Geometry: final body of the model. Coordinates: model frame, mm. A direction names the side the tool comes from. Round coordinates to 2 decimals unless told otherwise and drop trailing zeros. Loops run counter-clockwise (first coordinate to the right, second up) from the corner with the lowest first, then second, coordinate; pieces in that order, holes last. Notation, with made-up numbers: (86.25, 66.5) - (114.25, 66.5) arc R10 cw to (114.25, 70.5) - close; hole circle Ø7 at (78, 5.5). An arc over 180 degrees is marked (long way). Answer as a JSON object with one key per item and string values. Group by question number.
Item 1: Section A-A (z = 30.5). Return the cut outline in (x, y).
Item 2: Line query: line 1 (Y direction, x = 56, z = 1); line 2 (X direction, y = -19.5, z = 27.5); line 3 (Z direction, x = 37, y = 18.5). Output: solid intervals per line, ascending.
Item 3: Reachability of faces 5 (the face through (45, 0, 24)), 6 (the face through (-45, 0, 24)), 7 (the face through (40, 0, 24)) from +Z, -Z, +X, -X, +Y, -Y: full face, straight path, thin tool, end or side. Return the list, or none.
Item 4: Section B-B (x = 56.25). Return the cut outline in (y, z).
Item 5: Section D-D (y = -2.5). Return the cut outline in (x, z), plus the area to 3 significant figures.
Item 6: First-contact query: pin 1 (1 mm diameter, centred on x = 36.5, y = -1, fed in from +Z); pin 2 (4 mm diameter, centred on y = -10.5, z = 26.5, fed in from +X); pin 3 (6 mm diameter, centred on y = 4.5, z = 9.5, fed in from -X). Flat tips, straight axial feed; report the tip coordinate or a pass-through.
Item 7: Section C-C (y = 15). Return the cut outline in (x, z), plus the area to 3 significant figures.
Item 8: Draft query along Y for faces 1 (the face through (0, -22.5, 2)), 2 (the face through (-59, 0, 4)), 3 (the face through (0, 22.5, 2)), 4 (the face through (-59.3, 14.9, 2)). Return one class per face: released by +Y, released by -Y, zero draft, split by the parting line, or undercut.
Autodesk Inventor part; units mm, degrees
ref_plane "YZ Plane" through (0, 0, 0) normal (1, 0, 0) x (0, 1, 0)
ref_plane "XZ Plane" through (0, 0, 0) normal (0, 1, 0) x (-1, 0, 0)
ref_plane "XY Plane" through (0, 0, 0) normal (0, 0, 1) x (1, 0, 0)
sketch "Sketch1" plane through (0, 0, 0) normal (0, 0, 1) x (1, 0, 0)
  line L0 (-56.25, -15) -> (56.25, -15) construction
  line L1 (56.25, -15) -> (56.25, 15) construction
  line L2 (56.25, 15) -> (-56.25, 15) construction
  line L3 (-56.25, 15) -> (-56.25, -15) construction
  line L4 (-56.25, -15) -> (56.25, 15) construction
  line L5 (56.25, -15) -> (-56.25, 15) construction
  circle A0 centre (-56.25, 15) radius 3.05
  circle A1 centre (56.25, 15) radius 3.05
  circle A2 centre (56.25, -15) radius 3.05
  circle A3 centre (-56.25, -15) radius 3.05
  line L6 (-72.5, -22.5) -> (72.5, -22.5)
  line L7 (72.5, -22.5) -> (72.5, 22.5)
  line L8 (72.5, 22.5) -> (-72.5, 22.5)
  line L9 (-72.5, 22.5) -> (-72.5, -22.5)
  line L10 (-72.5, -22.5) -> (72.5, 22.5) construction
  line L11 (72.5, -22.5) -> (-72.5, 22.5) construction
  point P0 (0, 0)
  dimension "d0" = 112.5
  dimension "d1" = 30
  dimension "d2" = 6.1
  dimension "d3" = 145
  dimension "d4" = 45
extrude "Extrusion1" add sketch "Sketch1" along normal blind 4
sketch "Sketch2" plane through (0, 0, 4) normal (0, 0, 1) x (1, 0, 0)
  line L0 (72.5, 22.5) -> (-72.5, 22.5)
  line L1 (-72.5, -22.5) -> (72.5, -22.5)
  line L2 (-45, 22.5) -> (-40, 22.5)
  line L3 (-40, 22.5) -> (-40, -22.5)
  line L4 (-40, -22.5) -> (-45, -22.5)
  line L5 (-45, -22.5) -> (-45, 22.5)
  line L6 (40, 22.5) -> (45, 22.5)
  line L7 (45, 22.5) -> (45, -22.5)
  line L8 (45, -22.5) -> (40, -22.5)
  line L9 (40, -22.5) -> (40, 22.5)
  line L10 (-72.5, 22.5) -> (-72.5, -22.5)
  point P0 (0, 0)
  dimension "d7" = 5
  dimension "d8" = 5
  dimension "d9" = 80
  dimension "d10" = 27.5
extrude "Extrusion2" add sketch "Sketch2" along normal blind 40 contours L7 L1 L9 L0 | L3 L1 L5 L0
properties part number "WheelModuleBracket" material "ABS Plastic"
Values:
{
 "1": {"outline": "(-45, -22.5) - (-40, -22.5) - (-40, 22.5) - (-45, 22.5) - close; (40, -22.5) - (45, -22.5) - (45, 22.5) - (40, 22.5) - close"},
 "2": {"line 1": "y = -22.5 to -18.04, -11.96 to 11.96, 18.04 to 22.5", "line 2": "x = -45 to -40, 40 to 45", "line 3": "z = 0 to 4"},
 "3": {"face 5": "+Z, +X, +Y, -Y", "face 6": "+Z, -X, +Y, -Y", "face 7": "+Z, +Y, -Y"},
 "4": {"outline": "(-22.5, 0) - (-18.05, 0) - (-18.05, 4) - (-22.5, 4) - close; (-11.95, 0) - (11.95, 0) - (11.95, 4) - (-11.95, 4) - close; (18.05, 0) - (22.5, 0) - (22.5, 4) - (18.05, 4) - close"},
 "5": {"outline": "(-72.5, 0) - (72.5, 0) - (72.5, 4) - (45, 4) - (45, 44) - (40, 44) - (40, 4) - (-40, 4) - (-40, 44) - (-45, 44) - (-45, 4) - (-72.5, 4) - close", "area": "980 mm^2"},
 "6": {"pin 1": "stops at z = 4", "pin 2": "stops at x = 45", "pin 3": "stops at x = -45"},
 "7": {"outline": "(-72.5, 0) - (-59.3, 0) - (-59.3, 4) - (-72.5, 4) - close; (-53.2, 0) - (53.2, 0) - (53.2, 4) - (45, 4) - (45, 44) - (40, 44) - (40, 4) - (-40, 4) - (-40, 44) - (-45, 44) - (-45, 4) - (-53.2, 4) - close; (59.3, 0) - (72.5, 0) - (72.5, 4) - (59.3, 4) - close", "area": "931 mm^2"},
 "8": {"face 1": "released by -Y", "face 2": "zero draft", "face 3": "released by +Y", "face 4": "undercut"}
}
